Geometry check sheet. Reference: the model listing, model coordinates, mm. Face numbers are marked on the shaded views. A direction names the side the tool comes from. Round coordinates to 2 decimals unless told otherwise and drop trailing zeros. Write each loop counter-clockwise with the first axis right and the second up, starting at its lowest first coordinate (ties: lowest second). Pieces come first, ordered by that corner, then holes. Notation, with made-up numbers: M -15.75,83 L 18.25,83 A21 cw 18.25,119 Z; hole C 12.25,66.25 d7. An arc over 180 degrees is marked long. Answer in a Markdown table with one row per item. Add a question column.
from build123d import *

# Parameters (mm, degrees)
SKETCH_1_W          = 55
SKETCH_1_H          = 19.1
EXTRUDE_1_DEPTH     = 4
SKETCH_2_W          = 55
SKETCH_2_H          = 3.95
EXTRUDE_2_DEPTH     = 15.05
EXTRUDE_3_DEPTH     = 4
SKETCH_4_W          = 3.95
SKETCH_4_H          = 16.05
SKETCH_4_W_2        = 16
SKETCH_4_H_2        = 3.95
EXTRUDE_4_DEPTH     = 15.05
SKETCH_5_W          = 23
SKETCH_5_H          = 20
EXTRUDE_5_DEPTH     = 3.95
SKETCH_6_R          = 1.5
CUT_EXTRUDE_1_DEPTH = 4
SKETCH_7_R          = 1.5
SKETCH_7_R_2        = 1.78505628
CUT_EXTRUDE_2_DEPTH = 4


with BuildPart() as part:
    # Sketch 1 → Extrude 1 (new body)
    with BuildSketch(Plane(origin=(0, 0, 0), x_dir=(1, 0, 0), z_dir=(0, 1, 0))):
        with Locations((-13.411439114, 8.064760148)):
            Rectangle(SKETCH_1_W, SKETCH_1_H)
    extrude(amount=EXTRUDE_1_DEPTH)

    # Sketch 2 → Extrude 2 (add)
    with BuildSketch(Plane(origin=(0, 4, 0), x_dir=(1, 0, 0), z_dir=(0, 1, 0))):
        with Locations((-13.411439114, 15.639760148)):
            Rectangle(SKETCH_2_W, SKETCH_2_H)
    extrude(amount=EXTRUDE_2_DEPTH)



with BuildPart() as body_2:
    # Sketch 3 → Extrude 3 (new body)
    with BuildSketch(Plane.XZ):
        Polygon((-40.911439114, 5.435239852), (-40.911439114, 1.485239852), (-28.911439114, 1.485239852), (-5.911439114, 1.485239852), (14.088560886, 1.485239852), (14.088560886, 5.435239852), (-1.911439114, 5.435239852), (-1.911439114, 21.485239852), (-24.911439114, 21.485239852), (-24.911439114, 5.435239852), align=None)
    extrude(amount=-EXTRUDE_3_DEPTH)


with BuildPart() as part_1:
    add(part.part)

    add(body_2.part)  # Extrude 4 merges body 2
    # Sketch 4 → Extrude 4 (add)
    with BuildSketch(Plane(origin=(0, 4, 0), x_dir=(1, 0, 0), z_dir=(0, 1, 0))):
        with Locations((-3.886439114, -13.460239852)):
            Rectangle(SKETCH_4_W, SKETCH_4_H)
        Polygon((-1.911439114, -5.435239852), (14.088560886, -5.435239852), (14.088560886, -1.485239852), (-5.861439114, -1.485239852), (-5.861439114, -5.435239852), align=None)
        Polygon((-20.961439114, -21.485239852), (-20.961439114, -1.485239852), (-24.911439114, -1.485239852), (-24.911439114, -5.435239852), (-24.911439114, -21.485239852), align=None)
        with Locations((-32.911439114, -3.460239852)):
            Rectangle(SKETCH_4_W_2, SKETCH_4_H_2)
    extrude(amount=EXTRUDE_4_DEPTH)

    # Sketch 5 → Extrude 5 (add)
    with BuildSketch(Plane(origin=(0, 0, -17.614760148), x_dir=(-1, 0, 0), z_dir=(0, 0, -1))):
        with Locations((13.411439114, 29.05)):
            Rectangle(SKETCH_5_W, SKETCH_5_H)
    extrude(amount=-EXTRUDE_5_DEPTH)

    # Sketch 6 → Cut-Extrude 1 (cut)
    with BuildSketch(Plane(origin=(0, 0, -17.614760148), x_dir=(-1, 0, 0), z_dir=(0, 0, -1))):
        with Locations((13.411439114, 31.55)):
            Circle(SKETCH_6_R)
    extrude(amount=-CUT_EXTRUDE_1_DEPTH, mode=Mode.SUBTRACT)

    # Sketch 7 → Cut-Extrude 2 (cut)
    with BuildSketch(Plane.XZ):
        with Locations((6.588560886, -6.089760148)):
            Circle(SKETCH_7_R)
        with Locations((-33.411439114, -6.089760148)):
            Circle(SKETCH_7_R)
        with Locations((-13.411439114, 13.985239852)):
            Circle(SKETCH_7_R_2)
    extrude(amount=-CUT_EXTRUDE_2_DEPTH, mode=Mode.SUBTRACT)


solid = part_1.part
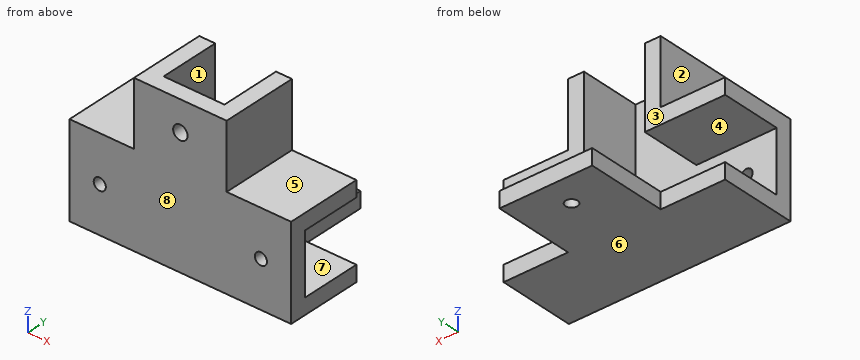
Item 1: Section check B-B, the plane x = -5. Record the boundary of the cut face in (y, z).
Item 2: Section check A-A, the plane y = 31.55. Record the boundary of the cut face in (x, z), and give its area (3 significant figures).
Item 3: Access from +Z, -Z, +X, -X, +Y, -Y to the whole of each face (thin tool, end or side, straight path). Record for the marked faces 1, 2, 3 and 4.
Item 4: Gauge pin test, flat ends, axial feed: pin 1 Ø10 at (x, z) = (8, 15) entering from +Y; pin 2 Ø16 at (x, z) = (-30.5, 15) entering from +Y; pin 3 Ø4 at (x, z) = (-33.41, -6.09) entering from +Y; pin 4 Ø8 at (x, y) = (9.5, 7) entering from +Z. Record the tip position at first contact, or that the pin passes through.
Item 5: Section check D-D, the plane z = 7. Record the boundary of the cut face in (x, y).
Item 6: Scan lines: probe 1 along X at (y, z) = (14.5, 17.5); probe 2 along Y at (x, z) = (-35, -12); probe 3 along Z at (x, y) = (-21.5, 23.5). Record each from-to range of solid material in increasing order. Write a range as from..to.
Item 7: Section check C-C, the plane y = 7.5. Record the boundary of the cut face in (x, z), and give its area (3 significant figures).
Item 8: Mould release check, pull along Z, two halves, no side actions. Record for the marked faces 5, 6, 7 and 8: +Z half, -Z half, draft (parallel to the pull), parting line (faces both ways), or undercut.
Result sheet:
| question | item | result |
|---|---|---|
| 1 | outline | M 0,-17.61 L 39.05,-17.61 L 39.05,-13.66 L 4,-13.66 L 4,1.49 L 19.05,1.49 L 19.05,21.49 L 0,21.49 Z |
| 2 | outline | M -24.91,-17.61 L -14.91,-17.61 L -14.91,-13.66 L -24.91,-13.66 Z; M -11.91,-17.61 L -1.91,-17.61 L -1.91,-13.66 L -11.91,-13.66 Z |
| 2 | area | 79.0 mm^2 |
| 3 | face 1 | +Z, +Y |
| 3 | face 2 | +Z, -X, +Y, -Y |
| 3 | face 3 | +Z, +X, -X, +Y |
| 3 | face 4 | +X, -X, +Y |
| 4 | pin 1 | passes through |
| 4 | pin 2 | stops at y = 19.05 |
| 4 | pin 3 | stops at y = 4 |
| 4 | pin 4 | stops at z = 5.44 |
| 5 | outline | M -24.91,0 L -1.91,0 L -1.91,19.05 L -5.86,19.05 L -5.86,4 L -20.96,4 L -20.96,19.05 L -24.91,19.05 Z |
| 6 | probe 1 | x = -24.91..-20.96, -5.86..-1.91 |
| 6 | probe 2 | y = 0..4 |
| 6 | probe 3 | z = -17.61..-13.66 |
| 7 | outline | M -40.91,-17.61 L 14.09,-17.61 L 14.09,-13.66 L -40.91,-13.66 Z; M -40.91,1.49 L -20.96,1.49 L -20.96,21.49 L -24.91,21.49 L -24.91,5.44 L -40.91,5.44 Z; M -5.86,1.49 L 14.09,1.49 L 14.09,5.44 L -1.91,5.44 L -1.91,21.49 L -5.86,21.49 Z |
| 7 | area | 502 mm^2 |
| 8 | face 5 | +Z half |
| 8 | face 6 | -Z half |
| 8 | face 7 | undercut |
| 8 | face 8 | draft |
